from build123d import *

# Parameters (mm, degrees)
F0_W     = 100
F0_H     = 50
F0_R     = 5
F1_DEPTH = 10
F2_R     = 1
F3_SIZE  = 1


with BuildPart() as f1:
    # F0 (on Front) → F1 (new body)
    with BuildSketch(Plane.XZ):
        Rectangle(F0_W, F0_H)
        with Locations((-30, -12.5)):
            Circle(F0_R, mode=Mode.SUBTRACT)
        with Locations((-30, 12.5)):
            Circle(F0_R, mode=Mode.SUBTRACT)
    extrude(amount=F1_DEPTH)

    # F2
    f2_edges = [f1.edges().sort_by_distance(p)[0] for p in [
        (50, -5, -25),
        (-50, -5, -25),
        (-50, -5, 25),
        (50, -5, 25),
    ]]
    fillet(f2_edges, radius=F2_R)

    # F3
    f3_edges = [f1.edges().sort_by_distance(p)[0] for p in [
        (50, -10, 0),
        (0, -10, -25),
        (-50, -10, 0),
        (0, -10, 25),
    ]]
    chamfer(f3_edges, length=F3_SIZE)


solid = f1.part
Can you work these out from the model? Positions are in its coordinate system, mm. Coordinates: 2 decimals unless noted, no trailing zeros. Write each loop counter-clockwise with the first axis right and the second up, starting at its lowest first coordinate (ties: lowest second). Pieces come first, ordered by that corner, then holes. Notation, with made-up numbers: (-0.75, 20.25) -> (45.25, 20.25) arc R23 cw to (45.25, 52.25) -> close; hole circle Ø9 at (88.25, -17). An arc over 180 degrees is marked (long way). Answer as CSV lines item,"result".
1) Will this pin go through, and if not, where does the flat tip stop? P1, Ø8, axis at x = -30, z = -12.5, coming from the +Y side.
Check result:
P1,"through"
2) If we section it at B-B on y = -1.5: Please give me the cut outline in (x, z), then the cut area to 3 significant figures.
Check result:
outline,"(-50, -24) arc R1 ccw to (-49, -25) -> (49, -25) arc R1 ccw to (50, -24) -> (50, 24) arc R1 ccw to (49, 25) -> (-49, 25) arc R1 ccw to (-50, 24) -> close; hole circle Ø10 at (-30, -12.5); hole circle Ø10 at (-30, 12.5)"
area,"4,840 mm²"
3) If we section it at C-C on z = 12.5: Please give me the cut outline in (x, y).
Check result:
outline,"(-50, -9) -> (-49, -10) -> (-35, -10) -> (-35, 0) -> (-50, 0) -> close; (-25, -10) -> (49, -10) -> (50, -9) -> (50, 0) -> (-25, 0) -> close"
4) If we mould it in two halves opening along Z, with no side actions, what happens to faces 1 (the flat face through (-1, -4, -25)), 2 (the cylindrical face through (-34.995, -4.93, -12.28)), 3 (the flat face through (-1, 0, 0))? For each: +Z half, -Z half, draft (parallel to the pull), parting line (faces both ways), or undercut.
Check result:
face 1,"-Z half"
face 2,"undercut"
face 3,"draft"
5) If I drill on line 1 (Z direction, x = -30, y = -6.25); line 2 (X direction, y = -3.5, z = 15.5); line 3 (Z direction, x = -26, y = -3.5), over which ranges is the centre line in solid material (lowest first)? Write a range as from..to.
Check result:
line 1,"-25..-17.5, -7.5..7.5, 17.5..25"
line 2,"-50..-34, -26..50"
line 3,"-25..-15.5, -9.5..9.5, 15.5..25"
6) If we section it at A-A on x = -30: Please give me the cut outline in (y, z), then the cut area to 3 significant figures.
Check result:
outline,"(-10, -24) -> (-9, -25) -> (0, -25) -> (0, -17.5) -> (-10, -17.5) -> close; (-10, -7.5) -> (0, -7.5) -> (0, 7.5) -> (-10, 7.5) -> close; (-10, 17.5) -> (0, 17.5) -> (0, 25) -> (-9, 25) -> (-10, 24) -> close"
area,"299 mm²"
